Answer from the drawing. Dimensions are ordinates in mm from the lowest x, y and z of the part. A direction names the side the tool comes from. Round coordinates to 2 decimals unless told otherwise and drop trailing zeros. Order: outer loops, then holes, each group sorted by start corner. A loop starts at its lowest first (then second) coordinate and runs counter-clockwise, first axis right, second up. Notation, with made-up numbers: M 40.25,-27.75 L 87.25,-27.75 A28 cw 87.25,-9.75 Z; hole C 47.25,37.25 d10. An arc over 180 degrees is marked long. Answer as a JSON object with one key per item and string values. Group by question number.
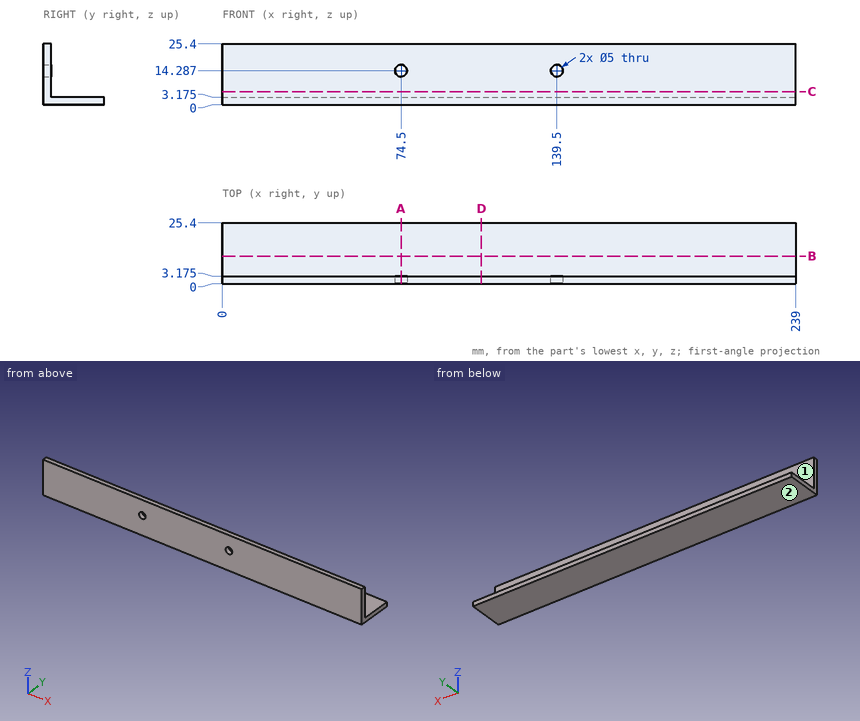
Item 1: A tool of negligible diameter and unlimited length cuts with its end or side. For the marked faces 1 and 2, from which of +Z, -Z, +X, -X, +Y, -Y can it reach the whole face along a straight path? Write none if from no direction.
Item 2: Find section B-B (y = 11.5). Give the vertices of the cut face in (x, z) (1 decimal).
Item 3: Consider L1, parallel to X at y = 1.5, z = 14.25; L2, parallel to Z at x = 139.5, y = 0.85; L3, parallel to Y at x = 84, z = 11.75 (1 decimal). Determine where each line is inside the solid, lowest interval first.
Item 4: Find section D-D (x = 108). Give the vertices of the cut face in (y, z) (1 decimal).
Item 5: Each of these flat-tipped pins is pushed along its axis until it touches: pin 1 (1.5 mm diameter, centred on x = 90.5, z = 10, fed in from +Y) (1 decimal); pin 2 (6.5 mm diameter, centred on x = 74.5, z = 14.29, fed in from -Y); pin 3 (11 mm diameter, centred on x = 76.5, y = 19, fed in from +Z) (1 decimal). Where does it stop, or does it pass through?
Item 6: Find section A-A (x = 74.5). Give the vertices of the cut face in (y, z) (1 decimal), and give its area (3 significant figures).
Responses:
{
 "1": {"face 1": "+Z, +X, -X, +Y", "face 2": "-Z, +X, -X, +Y, -Y"},
 "2": {"outline": "M 0,0 L 239,0 L 239,3.2 L 0,3.2 Z"},
 "3": {"L1": "x = 0 to 72, 77 to 137, 142 to 239", "L2": "z = 0 to 11.79, 16.79 to 25.4", "L3": "y = 0 to 3.2"},
 "4": {"outline": "M 0,0 L 25.4,0 L 25.4,3.2 L 3.2,3.2 L 3.2,25.4 L 0,25.4 Z"},
 "5": {"pin 1": "stops at y = 3.2", "pin 2": "stops at y = 0", "pin 3": "stops at z = 3.2"},
 "6": {"outline": "M 0,0 L 25.4,0 L 25.4,3.2 L 3.2,3.2 L 3.2,11.8 L 0,11.8 Z; M 0,16.8 L 3.2,16.8 L 3.2,25.4 L 0,25.4 Z", "area": "135 mm^2"}
}
